Input: part model. Units: mm. Frame: model coordinates. Face numbers are marked on the shaded views. Give positions to 0.01 mm unless a question says otherwise; leave off trailing zeros. Write each loop counter-clockwise with the first axis right and the second up, starting at its lowest first coordinate (ties: lowest second). Pieces come first, ordered by that corner, then holes.
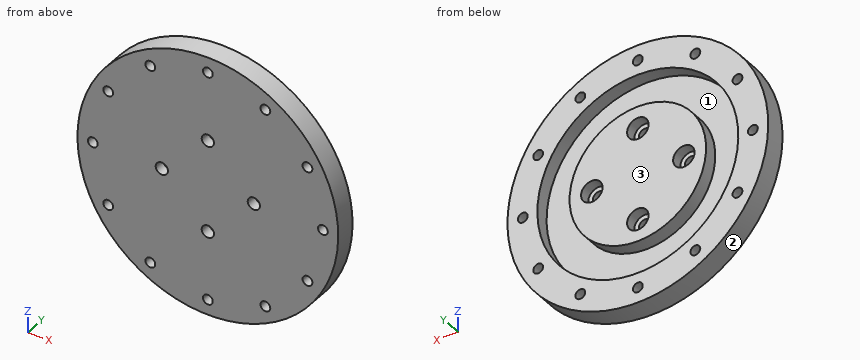
```python
from build123d import *

# Parameters (mm, degrees)
SKETCH1_R           = 42.5
BOSS_EXTRUDE1_DEPTH = 7
SKETCH2_R           = 32.75
SKETCH2_R_2         = 22.25
CUT_EXTRUDE1_DEPTH  = 4.5
SKETCH3_R           = 1.6
CUT_EXTRUDE2_DEPTH  = 61.510329697
SKETCH4_R           = 2
CUT_EXTRUDE3_DEPTH  = 61.510329697
SKETCH5_R           = 3.5
SKETCH5_R_2         = 2
CUT_EXTRUDE4_DEPTH  = 3.5


with BuildPart() as part:
    # Sketch1 → Boss-Extrude1 (new body)
    with BuildSketch(Plane(origin=(0, 0, 0), x_dir=(1, 0, 0), z_dir=(0, 1, 0))):
        with Locations(Location((0, 0, 0), (0, 0, 270))):
            Circle(SKETCH1_R)
    extrude(amount=BOSS_EXTRUDE1_DEPTH)

    # Sketch2 → Cut-Extrude1 (cut)
    with BuildSketch(Plane(origin=(0, 7, 0), x_dir=(1, 0, 0), z_dir=(0, 1, 0))):
        with Locations(Location((0, 0, 0), (0, 0, 270))):
            Circle(SKETCH2_R)
        with Locations(Location((0, 0, 0), (0, 0, 270))):
            Circle(SKETCH2_R_2, mode=Mode.SUBTRACT)
    extrude(amount=-CUT_EXTRUDE1_DEPTH, mode=Mode.SUBTRACT)

    # Sketch3 → Cut-Extrude2 (cut, through all)
    with BuildSketch(Plane(origin=(0, 7, 0), x_dir=(1, 0, 0), z_dir=(0, 1, 0))):
        with Locations(Location((0, 37.5, 0), (0, 0, 270))):
            Circle(SKETCH3_R)
        with Locations(Location((18.75, 32.475952642, 0), (0, 0, 270))):
            Circle(SKETCH3_R)
        with Locations(Location((32.475952642, 18.75, 0), (0, 0, 270))):
            Circle(SKETCH3_R)
        with Locations(Location((37.5, 0, 0), (0, 0, 270))):
            Circle(SKETCH3_R)
        with Locations(Location((32.475952642, -18.75, 0), (0, 0, 270))):
            Circle(SKETCH3_R)
        with Locations(Location((18.75, -32.475952642, 0), (0, 0, 270))):
            Circle(SKETCH3_R)
        with Locations(Location((0, -37.5, 0), (0, 0, 270))):
            Circle(SKETCH3_R)
        with Locations(Location((-18.75, -32.475952642, 0), (0, 0, 270))):
            Circle(SKETCH3_R)
        with Locations(Location((-32.475952642, -18.75, 0), (0, 0, 270))):
            Circle(SKETCH3_R)
        with Locations(Location((-37.5, 0, 0), (0, 0, 270))):
            Circle(SKETCH3_R)
        with Locations(Location((-32.475952642, 18.75, 0), (0, 0, 270))):
            Circle(SKETCH3_R)
        with Locations(Location((-18.75, 32.475952642, 0), (0, 0, 270))):
            Circle(SKETCH3_R)
    extrude(amount=-CUT_EXTRUDE2_DEPTH, mode=Mode.SUBTRACT)

    # Sketch4 → Cut-Extrude3 (cut, through all)
    with BuildSketch(Plane(origin=(0, 7, 0), x_dir=(1, 0, 0), z_dir=(0, 1, 0))):
        with Locations(Location((0, 15, 0), (0, 0, 270))):
            Circle(SKETCH4_R)
        with Locations(Location((15, 0, 0), (0, 0, 270))):
            Circle(SKETCH4_R)
        with Locations(Location((0, -15, 0), (0, 0, 270))):
            Circle(SKETCH4_R)
        with Locations(Location((-15, 0, 0), (0, 0, 270))):
            Circle(SKETCH4_R)
    extrude(amount=-CUT_EXTRUDE3_DEPTH, mode=Mode.SUBTRACT)

    # Sketch5 → Cut-Extrude4 (cut)
    # profile 1 of 4: a face of its own
    with BuildSketch(Plane(origin=(0, 7, 0), x_dir=(1, 0, 0), z_dir=(0, 1, 0))):
        with Locations(Location((0, 15, 0), (0, 0, 270))):
            Circle(SKETCH5_R)
        with Locations(Location((0, 15, 0), (0, 0, 270))):
            Circle(SKETCH5_R_2, mode=Mode.SUBTRACT)
    # profile 2 of 4: a face of its own
    with BuildSketch(Plane(origin=(0, 7, 0), x_dir=(1, 0, 0), z_dir=(0, 1, 0))):
        with Locations(Location((15, 0, 0), (0, 0, 270))):
            Circle(SKETCH5_R)
    # profile 3 of 4: a face of its own
    with BuildSketch(Plane(origin=(0, 7, 0), x_dir=(1, 0, 0), z_dir=(0, 1, 0))):
        with Locations(Location((0, -15, 0), (0, 0, 270))):
            Circle(SKETCH5_R)
    # profile 4 of 4: a face of its own
    with BuildSketch(Plane(origin=(0, 7, 0), x_dir=(1, 0, 0), z_dir=(0, 1, 0))):
        with Locations(Location((-15, 0, 0), (0, 0, 270))):
            Circle(SKETCH5_R)
    extrude(amount=-CUT_EXTRUDE4_DEPTH, mode=Mode.SUBTRACT)


solid = part.part
```
Item 1: Section B-B (z = -37.5). Return loops of the section in (x, y), and give its area (3 significant figures).
Item 2: Pin query (flat end, axial travel): pin 1 (4 mm diameter, centred on x = 22, y = 1, fed in from -Z); pin 2 (3 mm diameter, centred on x = -18.75, z = -32.48, fed in from -Y); pin 3 (4 mm diameter, centred on x = 22.5, y = 1.5, fed in from +Z); pin 4 (4 mm diameter, centred on x = 14, y = 3, fed in from +Z). Return the tip coordinate at first contact, or that it passes through.
Item 3: Ray query, line 1 (X direction, y = 6, z = 19); line 2 (Z direction, x = 16.5, y = 3); line 3 (Y direction, x = -8.5, z = -25). Return the intervals inside material, ascending.
Item 4: Section A-A (x = 37.5). Return loops of the section in (y, z).
Item 5: Section C-C (y = 5.75). Give the number of separate pieces and of enclosed holes in the cut face, and give its area (3 significant figures).
Item 6: Mould query, pull axis X, two halves, no side actions, for the marked faces 1, 2 and 3. Classes: +X half, -X half, draft (parallel to the pull), parting line (faces both ways), or undercut.
Solved:
1. outline: (-20, 0) - (-1.6, 0) - (-1.6, 7) - (-20, 7) - close; (1.6, 0) - (20, 0) - (20, 7) - (1.6, 7) - close
1. area: 258 mm2
2. pin 1: stops at z = -37.5
2. pin 2: passes through
2. pin 3: stops at z = 37.23
2. pin 4: stops at z = 40.77
3. line 1: x = -38.02 to -34.06, -30.9 to -26.68, -11.58 to 11.58, 26.68 to 30.9, 34.06 to 38.02
3. line 2: z = -39.17 to -28.29, -14.93 to -1.32, 1.32 to 14.93, 28.29 to 39.17
3. line 3: y = 0 to 2.5
4. outline: (0, -20) - (7, -20) - (7, -1.6) - (0, -1.6) - close; (0, 1.6) - (7, 1.6) - (7, 20) - (0, 20) - close
5. separate pieces: 2
5. enclosed holes: 17
5. area: 3,610 mm2
6. face 1: undercut
6. face 2: parting line
6. face 3: draft
